from build123d import *

# Parameters (mm, degrees)
F0_W     = 25.4
F0_H     = 57.15
F1_DEPTH = 12.7
F2_R     = 3.175
F3_DEPTH = 30.8102
F4_R     = 3.9624
F5_DEPTH = 41.40454
F6_R     = 1.0414
F7_DEPTH = 16.9418


with BuildPart() as f1:
    # F0 (on Top) → F1 (new body)
    with BuildSketch(Plane.XY):
        Rectangle(F0_W, F0_H)
    extrude(amount=F1_DEPTH)

    # F2 (on face) → F3 (cut)
    with BuildSketch(Plane(origin=(-12.7, 0, 0), x_dir=(0, -1, 0), z_dir=(-1, 0, 0))):
        with Locations((21.1582, 6.35)):
            Circle(F2_R)
    extrude(amount=-F3_DEPTH, mode=Mode.SUBTRACT)

    # F4 (on face) → F5 (cut)
    with BuildSketch(Plane(origin=(0, 28.575, 0), x_dir=(-1, 0, 0), z_dir=(0, 1, 0))):
        with Locations((6.35, 6.35)):
            Circle(F4_R)
    extrude(amount=-F5_DEPTH, mode=Mode.SUBTRACT)

    # F6 (on face) → F7 (cut)
    with BuildSketch(Plane.YZ.offset(12.7)):
        with Locations((-7.366, 6.121051)):
            Circle(F6_R)
    extrude(amount=-F7_DEPTH, mode=Mode.SUBTRACT)


solid = f1.part
Here's how the part is built. I have some questions about the finished solid (model axes, mm). A direction names the side the tool comes from. Coordinates: 2 decimals unless noted, no trailing zeros. Write each loop counter-clockwise with the first axis right and the second up, starting at its lowest first coordinate (ties: lowest second). Pieces come first, ordered by that corner, then holes.
1) I'm going to push flat-ended pins straight in: pin 1 (6.5 mm diameter, centred on x = -6.35, z = 6.35, fed in from +Y); pin 2 (1.7 mm diameter, centred on y = -7.37, z = 6.12, fed in from +X). Where does each tip first touch, or does it pass through?
Filled in:
pin 1: stops at y = -12.83
pin 2: stops at x = -10.16
2) If we section it at A-A (x = -6.35): List the corners of the cut face in (y, z) for me (3 decimals).
Filled in:
outline: (-28.575, 0) - (28.575, 0) - (28.575, 2.388) - (-12.83, 2.388) - (-12.83, 10.312) - (28.575, 10.312) - (28.575, 12.7) - (-28.575, 12.7) - close; hole circle Ø6.35 at (-21.158, 6.35)
3) Thinking about a two-plate mould opening in Z: for faces 4 (the face through (0, 0, 0)), 5 (the face through (-0.178, -24.187, 7.304)), 6 (the face through (-12.7, 0, 6)), which applies, +Z half, -Z half, draft (parallel to the pull), parting line (faces both ways), or undercut?
Filled in:
face 4: -Z half
face 5: undercut
face 6: draft
4) Which directions (+Z, -Z, +X, -X, +Y, -Y) give clear straight access to the entire face, cutting with the end or side of a thin tool? Please do faces 1 (the face through (0, 28.575, 6)), 2 (the face through (5.16, -6.37, 6.43)), 3 (the face through (-5.491, 8.163, 2.482)).
Filled in:
face 1: +Z, -Z, +X, -X, +Y
face 2: +X
face 3: +Y
5) If we section it at C-C (y = -12): List the corners of the cut face in (x, z) for me, plus the area to 3 significant figures.
Filled in:
outline: (-12.7, 0) - (12.7, 0) - (12.7, 12.7) - (-12.7, 12.7) - close; hole circle Ø7.92 at (-6.35, 6.35)
area: 273 mm2
6) If we section it at B-B (z = 7.75): List the corners of the cut face in (x, y) for me (3 decimals), plus the area to 4 significant figures.
Filled in:
outline: (-12.7, -28.575) - (12.7, -28.575) - (12.7, -24.008) - (-12.7, -24.008) - close; (-12.7, -18.309) - (12.7, -18.309) - (12.7, 28.575) - (-2.643, 28.575) - (-2.643, -12.83) - (-10.057, -12.83) - (-10.057, 28.575) - (-12.7, 28.575) - close
area: 1,000 mm2
7) If I drill on line 1 (Z direction, x = 4.25, y = -21); line 2 (X direction, y = 8, z = 6.35); line 3 (Z direction, x = -6.35, y = 14), over which ranges is the centre line in solid material (lowest first)?
Filled in:
line 1: z = 0 to 3.18, 9.52 to 12.7
line 2: x = -12.7 to -10.31, -2.39 to 12.7
line 3: z = 0 to 2.39, 10.31 to 12.7
8) If we section it at D-D (x = 6): List the corners of the cut face in (y, z) for me (3 decimals).
Filled in:
outline: (-28.575, 0) - (28.575, 0) - (28.575, 12.7) - (-28.575, 12.7) - close; hole circle Ø6.35 at (-21.158, 6.35); hole circle Ø2.083 at (-7.366, 6.121)
